from build123d import *

# Parameters (mm, degrees)
SKETCH1_W              = 1330
SKETCH1_H              = 100
BOSS_EXTRUDE1_DEPTH    = 30
BOSS_EXTRUDE1_2_DEPTH  = 30
BOSS_EXTRUDE1_3_DEPTH  = 30
BOSS_EXTRUDE1_4_DEPTH  = 30
BOSS_EXTRUDE1_5_DEPTH  = 30
BOSS_EXTRUDE1_6_DEPTH  = 30
BOSS_EXTRUDE1_7_DEPTH  = 30
BOSS_EXTRUDE1_8_DEPTH  = 30
BOSS_EXTRUDE1_9_DEPTH  = 30
BOSS_EXTRUDE1_10_DEPTH = 30
BOSS_EXTRUDE2_DEPTH    = 30


with BuildPart() as part:
    # Sketch1 → Boss-Extrude1 (new body)
    with BuildSketch(Plane.XY):
        with Locations((665, -500)):
            Rectangle(SKETCH1_W, SKETCH1_H)
    extrude(amount=BOSS_EXTRUDE1_DEPTH)



with BuildPart() as body_2:
    # Sketch1 → Boss-Extrude1 2 (new body)
    with BuildSketch(Plane.XY):
        with Locations((665, -700)):
            Rectangle(SKETCH1_W, SKETCH1_H)
    extrude(amount=BOSS_EXTRUDE1_2_DEPTH)


with BuildPart() as body_3:
    # Sketch1 → Boss-Extrude1 3 (new body)
    with BuildSketch(Plane.XY):
        with Locations((665, -900)):
            Rectangle(SKETCH1_W, SKETCH1_H)
    extrude(amount=BOSS_EXTRUDE1_3_DEPTH)


with BuildPart() as body_4:
    # Sketch1 → Boss-Extrude1 4 (new body)
    with BuildSketch(Plane.XY):
        with Locations((665, -1100)):
            Rectangle(SKETCH1_W, SKETCH1_H)
    extrude(amount=BOSS_EXTRUDE1_4_DEPTH)


with BuildPart() as body_5:
    # Sketch1 → Boss-Extrude1 5 (new body)
    with BuildSketch(Plane.XY):
        with Locations((665, -1300)):
            Rectangle(SKETCH1_W, SKETCH1_H)
    extrude(amount=BOSS_EXTRUDE1_5_DEPTH)


with BuildPart() as body_6:
    # Sketch1 → Boss-Extrude1 6 (new body)
    with BuildSketch(Plane.XY):
        with Locations((665, -1900)):
            Rectangle(SKETCH1_W, SKETCH1_H)
    extrude(amount=BOSS_EXTRUDE1_6_DEPTH)


with BuildPart() as body_7:
    # Sketch1 → Boss-Extrude1 7 (new body)
    with BuildSketch(Plane.XY):
        with Locations((665, -100)):
            Rectangle(SKETCH1_W, SKETCH1_H)
    extrude(amount=BOSS_EXTRUDE1_7_DEPTH)


with BuildPart() as body_8:
    # Sketch1 → Boss-Extrude1 8 (new body)
    with BuildSketch(Plane.XY):
        with Locations((665, -300)):
            Rectangle(SKETCH1_W, SKETCH1_H)
    extrude(amount=BOSS_EXTRUDE1_8_DEPTH)


with BuildPart() as body_9:
    # Sketch1 → Boss-Extrude1 9 (new body)
    with BuildSketch(Plane.XY):
        with Locations((665, -1500)):
            Rectangle(SKETCH1_W, SKETCH1_H)
    extrude(amount=BOSS_EXTRUDE1_9_DEPTH)


with BuildPart() as body_10:
    # Sketch1 → Boss-Extrude1 10 (new body)
    with BuildSketch(Plane.XY):
        with Locations((665, -1700)):
            Rectangle(SKETCH1_W, SKETCH1_H)
    extrude(amount=BOSS_EXTRUDE1_10_DEPTH)


with BuildPart() as part_1:
    add(part.part)

    add(body_2.part)  # Boss-Extrude2 merges body 2

    add(body_3.part)  # Boss-Extrude2 merges body 3

    add(body_4.part)  # Boss-Extrude2 merges body 4

    add(body_5.part)  # Boss-Extrude2 merges body 5

    add(body_6.part)  # Boss-Extrude2 merges body 6

    add(body_7.part)  # Boss-Extrude2 merges body 7

    add(body_8.part)  # Boss-Extrude2 merges body 8

    add(body_9.part)  # Boss-Extrude2 merges body 9

    add(body_10.part)  # Boss-Extrude2 merges body 10
    # Sketch2 → Boss-Extrude2 (add)
    with BuildSketch(Plane.XY.offset(30)):
        Polygon((1330, -50), (0, -1050), (0, -1150), (1330, -150), align=None)
        Polygon((1330, -850), (0, -1850), (0, -1950), (1330, -950), align=None)
    extrude(amount=BOSS_EXTRUDE2_DEPTH)


solid = part_1.part
Can you work these out from the model? Positions are in its coordinate system, mm. A direction names the side the tool comes from. Give positions to 0.01 mm unless a question says otherwise; leave off trailing zeros. Loops run counter-clockwise (first coordinate to the right, second up) from the corner with the lowest first, then second, coordinate; pieces in that order, holes last. Notation, with made-up numbers: M 25.25,-33 L 51.25,-33 A23 cw 51.25,-20 Z; hole C 25.5,55 d6. An arc over 180 degrees is marked long. One line per item, written item: value.
1) Imagine slicing it at A-A on z = 47.5. Write out the boundary of the cut face in (x, y), and give its area (3 significant figures).
Geometry check:
outline: M 0,-1950 L 1330,-950 L 1330,-850 L 0,-1850 Z; M 0,-1150 L 1330,-150 L 1330,-50 L 0,-1050 Z
area: 266,000 mm²
2) I'm going to push flat-ended pins straight in: pin 1 (3 mm diameter, centred on x = 589, z = 40, fed in from +Y); pin 2 (5 mm diameter, centred on x = 995, z = 48, fed in from +Y). Where does each tip first touch, or does it pass through?
Geometry check:
pin 1: stops at y = -606.02
pin 2: stops at y = -300
3) On a 3-axis mill with a long thin cutter (end or side, diameter ignored), from which of +Z, -Z, +X, -X, +Y, -Y can I reach the whole of each face in a straight line? I mean faces 4 (the face through (1225, -299, 30)), 5 (the face through (1330, -101, 30)), 6 (the face through (656, -99, 30)), 7 (the face through (663, -1399, 30)), 8 (the face through (1119, -1299, 30)). Say none if no direction works.
Geometry check:
face 4: +Z, +X
face 5: +Z, -Z, +X, +Y, -Y
face 6: +Z, -X, +Y
face 7: -Z, +X, -X
face 8: +Z, +X, -Y
4) Imagine slicing it at D-D on y = -222. Write out the boundary of the cut face in (x, z), and give its area (3 significant figures).
Geometry check:
outline: M 1101.24,30 L 1234.24,30 L 1234.24,60 L 1101.24,60 Z
area: 3,990 mm²
5) Thinking about a two-plate mould opening in Y: for faces 1 (the face through (674.31, -543, 44.79)), 2 (the face through (1195, -999, 30)), 3 (the face through (656, -99, 0)), which applies, +Y half, -Y half, draft (parallel to the pull), parting line (faces both ways), or undercut?
Geometry check:
face 1: +Y half
face 2: undercut
face 3: draft
6) Please list where these lines run through material, in increasing order: line 1 (Z direction, x = 112, y = -904); line 2 (Y direction, x = 274.5, z = 51); line 3 (Y direction, x = 933, z = 45.5).
Geometry check:
line 1: z = 0 to 30
line 2: y = -1743.61 to -1643.61, -943.61 to -843.61
line 3: y = -1248.5 to -1148.5, -448.5 to -348.5
7) Imagine slicing it at B-B on y = -1317. Write out the boundary of the cut face in (x, z), and give its area (3 significant figures).
Geometry check:
outline: M 0,0 L 1330,0 L 1330,30 L 841.89,30 L 841.89,60 L 708.89,60 L 708.89,30 L 0,30 Z
area: 43,900 mm²
8) Imagine slicing it at C-C on x = 568.5. Count the separate pieces of the cut face and the enclosed holes in it, and give its area (3 significant figures).
Geometry check:
separate pieces: 10
enclosed holes: 0
area: 36,000 mm²
